```python
from build123d import *
from build123d.topology import SkipClean

# Parameters (mm, degrees)
SKETCH_1_W          = 3.0000000000000027
SKETCH_1_H          = 26
EXTRUDE_1_DEPTH     = 21.2
EXTRUDE_2_DEPTH     = 3
SKETCH_2_R          = 14.3
CUT_EXTRUDE_1_DEPTH = 1
EXTRUDE_START       = 3
EXTRUDE_3_DEPTH     = 3
EXTRUDE_START_2     = 10
EXTRUDE_4_DEPTH     = 7
SKETCH_7_R          = 1.0000000000000018
SKETCH_7_R_2        = 1.0000000000000016
CUT_EXTRUDE_2_DEPTH = 42.41376582731883
SKETCH_7_3_R        = 1.5000000000000009
SKETCH_7_3_R_2      = 1.0000000000000018
SKETCH_7_3_R_3      = 1.5000000000000004
SKETCH_7_3_R_4      = 1.0000000000000016
CUT_EXTRUDE_3_DEPTH = 1
CUT_EXTRUDE_START   = -29.2
SKETCH_7_4_R        = 1.5000000000000009
SKETCH_7_4_R_2      = 1.0000000000000018
SKETCH_7_4_R_3      = 1.5000000000000004
SKETCH_7_4_R_4      = 1.0000000000000016
CUT_EXTRUDE_4_DEPTH = 1
OTHER_START         = -0.5
OTHER_1_OUTLINE_R   = 1
OTHER_1_DEPTH       = 2


# Read off the part's stored shape, not the designer's step: 填充阵列1
with BuildPart() as part:
    # 草图1 → 凸台-拉伸1 (new body)
    with BuildSketch(Plane(origin=(0, 0, 0), x_dir=(1, 0, 0), z_dir=(0, 1, 0))):
        Rectangle(SKETCH_1_W, SKETCH_1_H)
    extrude(amount=EXTRUDE_1_DEPTH)

    # 草图5 → 凸台-拉伸2 (add)
    with BuildSketch(Plane(origin=(1.5000000000000013, 0, 0), x_dir=(0, 0, -1), z_dir=(1, 0, 0))):
        Polygon((-15.100000000000001, 25.9), (15.099999999999998, 25.900000000000002), (15.100000000000001, -4.299999999999996), (-15.099999999999998, -4.3), align=None)
    extrude(amount=-EXTRUDE_2_DEPTH)

    # 草图2 → 切除-拉伸1 (cut)
    with BuildSketch(Plane.ZY.offset(1.5000000000000013)):
        with Locations((1.8546e-13, 10.35000000000003)):
            Circle(SKETCH_2_R)
    extrude(amount=-CUT_EXTRUDE_1_DEPTH, mode=Mode.SUBTRACT)

    # 草图6 → 凸台-拉伸3 (add)
    with SkipClean():  # the faces are left unmerged after this step: merging them gives an invalid solid
        with BuildSketch(Plane.ZY.offset(1.5000000000000013).offset(EXTRUDE_START)):
            with BuildLine():
                Line((15.100000000000001, 25.9), (-15.099999999999998, 25.9))
                Line((-15.099999999999998, 25.9), (-15.099999999999994, 21.4))
                Line((-15.099999999999994, 21.4), (-13.099999999999994, 21.4))
                Line((-13.099999999999994, 21.4), (-9.076756028450045, 21.4))
                ThreePointArc((-9.07675602844997, 21.39999999999975), (-2.1374e-13, 24.65000000000003), (9.076756028449726, 21.400000000000254))
                Line((9.076756028449651, 21.4), (13.100000000000001, 21.4))
                Line((13.100000000000001, 21.4), (15.100000000000001, 21.4))
                Line((15.100000000000001, 21.4), (15.100000000000001, 25.9))
            make_face()
            with BuildLine():
                Line((-13.099999999999994, 21.4), (-15.099999999999994, 21.4))
                Line((-15.099999999999994, 21.4), (-15.099999999999994, -4.3))
                Line((-15.099999999999994, -4.3), (-13.099999999999994, -4.3))
                Line((-13.099999999999994, -4.3), (-13.099999999999994, 4.615891525267789))
                ThreePointArc((-13.099999999999968, 4.615891525267795), (-14.299999999999816, 10.350000000000032), (-13.099999999999962, 16.084108474732275))
                Line((-13.099999999999994, 16.084108474732275), (-13.099999999999994, 21.4))
            make_face()
            with BuildLine():
                Line((-9.076756028450045, 21.4), (-13.099999999999994, 21.4))
                Line((-13.099999999999994, 21.4), (-13.099999999999994, 16.084108474732275))
                ThreePointArc((-13.099999999999962, 16.084108474732275), (-11.4024910727196, 18.979785474537948), (-9.07675602844997, 21.39999999999975))
            make_face()
            with BuildLine():
                Line((13.100000000000001, 16.084108474732616), (13.100000000000001, 21.4))
                Line((13.100000000000001, 21.4), (9.076756028449651, 21.4))
                ThreePointArc((9.076756028449726, 21.400000000000254), (11.402491072719606, 18.97978547453843), (13.100000000000168, 16.084108474732652))
            make_face()
            with BuildLine():
                Line((15.100000000000001, -4.3), (15.100000000000001, 21.4))
                Line((15.100000000000001, 21.4), (13.100000000000001, 21.4))
                Line((13.100000000000001, 21.4), (13.100000000000001, 16.084108474732616))
                ThreePointArc((13.100000000000168, 16.084108474732652), (13.996785345214274, 13.279163703175414), (14.300000000000185, 10.35000000000003))
                ThreePointArc((14.300000000000185, 10.350000000000026), (13.996785345214237, 7.420836296824469), (13.100000000000025, 4.615891525267081))
                Line((13.100000000000001, 4.6158915252670925), (13.100000000000001, -4.3))
                Line((13.100000000000001, -4.3), (15.100000000000001, -4.3))
            make_face()
            with BuildLine():
                Line((-13.099999999999994, 4.615891525267789), (-13.099999999999994, -4.3))
                Line((-13.099999999999994, -4.299999999999996), (13.100000000000001, -4.3))
                Line((13.100000000000001, -4.3), (13.100000000000001, 4.6158915252670925))
                ThreePointArc((13.100000000000025, 4.615891525267081), (-1.982e-13, -3.949999999999971), (-13.099999999999968, 4.615891525267795))
            make_face()
        extrude(amount=-EXTRUDE_3_DEPTH)

    # 草图6<3> → 凸台-拉伸4 (add)
    with BuildSketch(Plane.ZY.offset(1.5000000000000013).offset(EXTRUDE_START_2)):
        with BuildLine():
            Line((15.100000000000001, 25.9), (-15.099999999999998, 25.9))
            Line((-15.099999999999998, 25.9), (-15.099999999999994, 21.4))
            Line((-15.099999999999994, 21.4), (-13.099999999999994, 21.4))
            Line((-13.099999999999994, 21.4), (-9.076756028450045, 21.4))
            ThreePointArc((-9.07675602844997, 21.39999999999975), (-2.1374e-13, 24.65000000000003), (9.076756028449726, 21.400000000000254))
            Line((9.076756028449651, 21.4), (13.100000000000001, 21.4))
            Line((13.100000000000001, 21.4), (15.100000000000001, 21.4))
            Line((15.100000000000001, 21.4), (15.100000000000001, 25.9))
        make_face()
        with BuildLine():
            Line((-13.099999999999994, 21.4), (-15.099999999999994, 21.4))
            Line((-15.099999999999994, 21.4), (-15.099999999999994, -4.3))
            Line((-15.099999999999994, -4.3), (-13.099999999999994, -4.3))
            Line((-13.099999999999994, -4.3), (-13.099999999999994, 4.615891525267789))
            ThreePointArc((-13.099999999999968, 4.615891525267795), (-14.299999999999816, 10.350000000000032), (-13.099999999999962, 16.084108474732275))
            Line((-13.099999999999994, 16.084108474732275), (-13.099999999999994, 21.4))
        make_face()
        with BuildLine():
            Line((15.100000000000001, -4.3), (15.100000000000001, 21.4))
            Line((15.100000000000001, 21.4), (13.100000000000001, 21.4))
            Line((13.100000000000001, 21.4), (13.100000000000001, 16.084108474732616))
            ThreePointArc((13.100000000000168, 16.084108474732652), (13.996785345214274, 13.279163703175414), (14.300000000000185, 10.35000000000003))
            ThreePointArc((14.300000000000185, 10.350000000000026), (13.996785345214237, 7.420836296824469), (13.100000000000025, 4.615891525267081))
            Line((13.100000000000001, 4.6158915252670925), (13.100000000000001, -4.3))
            Line((13.100000000000001, -4.3), (15.100000000000001, -4.3))
        make_face()
    extrude(amount=-EXTRUDE_4_DEPTH)

    # 草图7 → 切除-拉伸2 (cut, through all)
    with BuildSketch(Plane(origin=(0, 1.73e-15, -15.100000000000001), x_dir=(-1, 0, 0), z_dir=(0, 1.1e-16, -1))):
        with Locations(Location((8.599999999999989, 18.2, 0), (0, 0, 90))):
            Circle(SKETCH_7_R)
        with Locations(Location((8.599999999999989, 3, 0), (0, 0, 90))):
            Circle(SKETCH_7_R_2)
    extrude(amount=-CUT_EXTRUDE_2_DEPTH, mode=Mode.SUBTRACT)

    # 草图7<3> → 切除-拉伸3 (cut)
    # profile 1 of 2: a face of its own
    with BuildSketch(Plane(origin=(0, 1.73e-15, -15.100000000000001), x_dir=(-1, 0, 0), z_dir=(0, 1.1e-16, -1))):
        with Locations(Location((8.599999999999989, 18.2, 0), (0, 0, 90))):
            Circle(SKETCH_7_3_R)
        with Locations(Location((8.599999999999989, 18.2, 0), (0, 0, 90))):
            Circle(SKETCH_7_3_R_2, mode=Mode.SUBTRACT)
    # profile 2 of 2: a face of its own
    with BuildSketch(Plane(origin=(0, 1.73e-15, -15.100000000000001), x_dir=(-1, 0, 0), z_dir=(0, 1.1e-16, -1))):
        with Locations(Location((8.599999999999989, 3, 0), (0, 0, 90))):
            Circle(SKETCH_7_3_R_3)
        with Locations(Location((8.599999999999989, 3, 0), (0, 0, 90))):
            Circle(SKETCH_7_3_R_4, mode=Mode.SUBTRACT)
    extrude(amount=-CUT_EXTRUDE_3_DEPTH, mode=Mode.SUBTRACT)

    # 草图7<4> → 切除-拉伸4 (cut)
    # profile 1 of 2: a face of its own
    with BuildSketch(Plane(origin=(0, 1.73e-15, -15.100000000000001), x_dir=(-1, 0, 0), z_dir=(0, 1.1e-16, -1)).offset(CUT_EXTRUDE_START)):
        with Locations(Location((8.599999999999989, 18.2, 0), (0, 0, 90))):
            Circle(SKETCH_7_4_R)
        with Locations(Location((8.599999999999989, 18.2, 0), (0, 0, 90))):
            Circle(SKETCH_7_4_R_2, mode=Mode.SUBTRACT)
    # profile 2 of 2: a face of its own
    with BuildSketch(Plane(origin=(0, 1.73e-15, -15.100000000000001), x_dir=(-1, 0, 0), z_dir=(0, 1.1e-16, -1)).offset(CUT_EXTRUDE_START)):
        with Locations(Location((8.599999999999989, 3, 0), (0, 0, 90))):
            Circle(SKETCH_7_4_R_3)
        with Locations(Location((8.599999999999989, 3, 0), (0, 0, 90))):
            Circle(SKETCH_7_4_R_4, mode=Mode.SUBTRACT)
    extrude(amount=-CUT_EXTRUDE_4_DEPTH, mode=Mode.SUBTRACT)

    # 填充阵列1 outline → 填充阵列1 (cut)
    with BuildSketch(Plane.YZ.offset(OTHER_START)):
        with Locations((10.35, -3.37e-06)):
            Circle(OTHER_1_OUTLINE_R)
        with Locations((10.35, -12.00000337)):
            Circle(OTHER_1_OUTLINE_R)
        with Locations((6.641796068, -11.412681566)):
            Circle(OTHER_1_OUTLINE_R)
        with Locations((3.296576972, -9.708207303)):
            Circle(OTHER_1_OUTLINE_R)
        with Locations((17.557750943, -3.471073283)):
            Circle(OTHER_1_OUTLINE_R)
        with Locations((14.058203932, -11.412681566)):
            Circle(OTHER_1_OUTLINE_R)
        with Locations((17.403423028, -9.708207303)):
            Circle(OTHER_1_OUTLINE_R)
        with Locations((20.058203932, -7.053426398)):
            Circle(OTHER_1_OUTLINE_R)
        with Locations((21.762678196, -3.708207303)):
            Circle(OTHER_1_OUTLINE_R)
        with Locations((17.403423028, 9.708200562)):
            Circle(OTHER_1_OUTLINE_R)
        with Locations((12.130167472, 7.799419927)):
            Circle(OTHER_1_OUTLINE_R)
        with Locations((6.35, -3.37e-06)):
            Circle(OTHER_1_OUTLINE_R)
        with Locations((20.058203932, 7.053419657)):
            Circle(OTHER_1_OUTLINE_R)
        with Locations((8.35, -3.464104985)):
            Circle(OTHER_1_OUTLINE_R)
        with Locations((8.569832528, 7.799419927)):
            Circle(OTHER_1_OUTLINE_R)
        with Locations((14.058203932, 11.412674825)):
            Circle(OTHER_1_OUTLINE_R)
        with Locations((12.35, -3.464104985)):
            Circle(OTHER_1_OUTLINE_R)
        with Locations((12.35, 3.464098245)):
            Circle(OTHER_1_OUTLINE_R)
        with Locations((22.35, -3.37e-06)):
            Circle(OTHER_1_OUTLINE_R)
        with Locations((18.35, -3.37e-06)):
            Circle(OTHER_1_OUTLINE_R)
        with Locations((14.35, -3.37e-06)):
            Circle(OTHER_1_OUTLINE_R)
        with Locations((17.557750943, 3.471066543)):
            Circle(OTHER_1_OUTLINE_R)
        with Locations((21.762678196, 3.708200562)):
            Circle(OTHER_1_OUTLINE_R)
        with Locations((8.35, 3.464098245)):
            Circle(OTHER_1_OUTLINE_R)
        with Locations((15.337918415, 6.25464849)):
            Circle(OTHER_1_OUTLINE_R)
        with Locations((-1.65, -3.37e-06)):
            Circle(OTHER_1_OUTLINE_R)
        with Locations((8.569832528, -7.799426668)):
            Circle(OTHER_1_OUTLINE_R)
        with Locations((-1.062678196, 3.708200562)):
            Circle(OTHER_1_OUTLINE_R)
        with Locations((5.362081585, -6.25465523)):
            Circle(OTHER_1_OUTLINE_R)
        with Locations((0.641796068, -7.053426398)):
            Circle(OTHER_1_OUTLINE_R)
        with Locations((15.337918415, -6.25465523)):
            Circle(OTHER_1_OUTLINE_R)
        with Locations((-1.062678196, -3.708207303)):
            Circle(OTHER_1_OUTLINE_R)
        with Locations((12.130167472, -7.799426668)):
            Circle(OTHER_1_OUTLINE_R)
        with Locations((6.641796068, 11.412674825)):
            Circle(OTHER_1_OUTLINE_R)
        with Locations((3.142249057, 3.471066543)):
            Circle(OTHER_1_OUTLINE_R)
        with Locations((10.35, 11.99999663)):
            Circle(OTHER_1_OUTLINE_R)
        with Locations((5.362081585, 6.25464849)):
            Circle(OTHER_1_OUTLINE_R)
        with Locations((0.641796068, 7.053419657)):
            Circle(OTHER_1_OUTLINE_R)
        with Locations((3.142249057, -3.471073283)):
            Circle(OTHER_1_OUTLINE_R)
        with Locations((3.296576972, 9.708200562)):
            Circle(OTHER_1_OUTLINE_R)
        with Locations((2.35, -3.37e-06)):
            Circle(OTHER_1_OUTLINE_R)
    extrude(amount=OTHER_1_DEPTH, mode=Mode.SUBTRACT)


solid = part.part
```
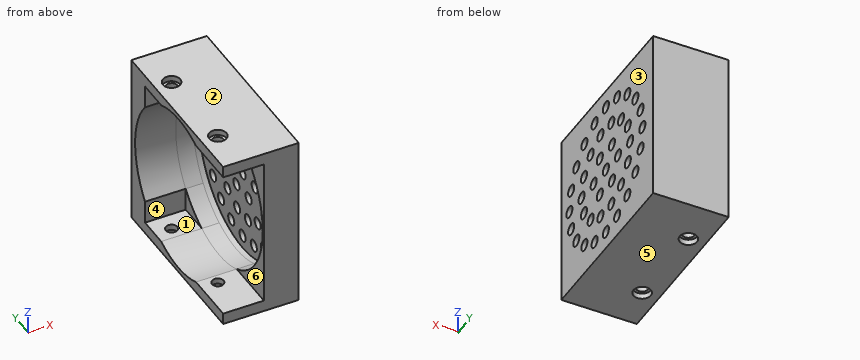
Input: part model. Units: mm. Frame: model coordinates. Face numbers are marked on the shaded views. A direction names the side the tool comes from. Round coordinates to 2 decimals unless told otherwise and drop trailing zeros. Write each loop counter-clockwise with the first axis right and the second up, starting at its lowest first coordinate (ties: lowest second). Pieces come first, ordered by that corner, then holes. Notation, with made-up numbers: M -8.5,-29 L -2.5,-29 A22 ccw -2.5,-18 Z; hole C 77,51 d1. An arc over 180 degrees is marked long. Write each question's results on one line, items separated by ' | '.
Q1. Line query: line 1 along Z through (x, y) = (-10.5, 19.5); line 2 along Z through (x, y) = (0.5, 5); line 3 along Y through (x, z) = (-7.75, 14.5). Output: solid intervals per line, ascending.
Results:
line 1: z = -15.1 to -13.1, 13.1 to 15.1 | line 2: z = -15.1 to -7.19, -5.32 to 5.32, 7.19 to 15.1 | line 3: y = -4.3 to 1.76, 4.24 to 16.96, 19.44 to 25.9
Q2. Section query C-C (y = 22.35). Return loops of the section in (x, z), and give its area (3 significant figures).
Results:
outline: M -11.5,-15.1 L 1.5,-15.1 L 1.5,-4.52 L -0.5,-4.52 L -0.5,-7.78 L -11.5,-7.78 Z; M -11.5,7.78 L -0.5,7.78 L -0.5,4.52 L 1.5,4.52 L 1.5,15.1 L -11.5,15.1 Z; M -0.5,-2.9 L 1.5,-2.9 L 1.5,-1 L -0.5,-1 Z; M -0.5,1 L 1.5,1 L 1.5,2.9 L -0.5,2.9 Z | area: 211 mm^2
Q3. Section query A-A (x = -2.25). Return loops of the section in (y, z).
Results:
outline: M -4.3,-15.1 L 25.9,-15.1 L 25.9,15.1 L -4.3,15.1 Z; hole C 10.35,0 d28.6
Q4. Pin query (flat end, axial travel): P1, Ø6, axis at y = 5, z = -6.5, coming from the -X side; P2, Ø1.5, axis at x = -9, y = 3, coming from the -Z side; P3, Ø1.2, axis at y = 19.5, z = -10.5, coming from the -X side; P4, Ø1.8, axis at x = -8.6, y = 3, coming from the -Z side. Return the tip coordinate at first contact, or that it passes through.
Results:
P1: stops at x = -0.5 | P2: stops at z = -14.1 | P3: stops at x = -4.5 | P4: passes through
Q5. Draft query along Z for the marked faces 3, 4, 5 and 6. Return one class per face: released by +Z, released by -Z, zero draft, split by the parting line, or undercut.
Results:
face 3: zero draft | face 4: undercut | face 5: released by -Z | face 6: undercut
Q6. Section query B-B (y = 12.35). Return loops of the section in (x, z).
Results:
outline: M -11.5,-15.1 L 1.5,-15.1 L 1.5,-8.77 L -0.5,-8.77 L -0.5,-14.16 L -11.5,-14.16 Z; M -11.5,14.16 L -0.5,14.16 L -0.5,8.77 L 1.5,8.77 L 1.5,15.1 L -11.5,15.1 Z; M -0.5,-6.82 L 1.5,-6.82 L 1.5,-4.46 L -0.5,-4.46 Z; M -0.5,-2.46 L 1.5,-2.46 L 1.5,2.46 L -0.5,2.46 Z; M -0.5,4.46 L 1.5,4.46 L 1.5,6.82 L -0.5,6.82 Z
Q7. Access query for the marked faces 1 and 2. Directions: +Z, -Z, +X, -X, +Y, -Y. A direction counts if a zero-diameter tool reaches every point of the face in a straight line with its end or side. Return the directions, or none.
Results:
face 1: -X, -Y | face 2: +Z, +X, -X, +Y, -Y
Q8. Section query D-D (x = -10.5). Return loops of the section in (y, z).
Results:
outline: M -4.3,-15.1 L 25.9,-15.1 L 25.9,15.1 L -4.3,15.1 L -4.3,13.1 L 4.62,13.1 A14.3 cw 16.08,13.1 L 21.4,13.1 L 21.4,9.08 A14.3 cw 21.4,-9.08 L 21.4,-13.1 L 16.08,-13.1 A14.3 cw 4.62,-13.1 L -4.3,-13.1 Z
